from build123d import *

# Parameters (mm, degrees)
F0_W     = 177.8
F0_H     = 292.1
F1_DEPTH = 12.7
F2_SIZE2 = 85.72499
F2_SIZE  = 292.09999


# Not quite as in the source:
# - a fillet or chamfer is up to 0.001 mm smaller than in the source, because OpenCascade refuses the exact size


with BuildPart() as f1:
    # F0 (on Front) → F1 (new body)
    with BuildSketch(Plane.XZ):
        Rectangle(F0_W, F0_H)
    extrude(amount=F1_DEPTH)

    # F2 (size 292.1 and 85.725 in the source; OpenCascade refuses exactly that, so slightly less here)
    f2_edges = [f1.edges().sort_by_distance(p)[0] for p in [
        (-88.9, -6.35, 146.05),
    ]]
    f2_side = f1.faces().sort_by_distance((-88.9, -6.35, 0))[0]
    chamfer(f2_edges, length=F2_SIZE, length2=F2_SIZE2, reference=f2_side)


solid = f1.part
Build history of the part. All positions in model axes, mm. Coordinates: 2 decimals unless noted, no trailing zeros. Write each loop counter-clockwise with the first axis right and the second up, starting at its lowest first coordinate (ties: lowest second). Pieces come first, ordered by that corner, then holes.
(1) Cut at B-B on z = 31.5. List the corners of the cut face in (x, y).
(2) Cut at C-C on x = -49. List the corners of the cut face in (y, z), and give its area (3 significant figures).
(3) Drill centre lines: line 1 (X direction, y = -5, z = 6.5); line 2 (X direction, y = -7.25, z = 100). Where is each one in solid material? Low to high.
Working result:
1. outline: (-36.79, -12.7) - (88.9, -12.7) - (88.9, 0) - (-36.79, 0) - close
2. outline: (-12.7, -146.05) - (0, -146.05) - (0, -10.09) - (-12.7, -10.09) - close
2. area: 1,730 mm2
3. line 1: x = -44.13 to 88.9
3. line 2: x = -16.69 to 88.9
